Here's the drawing with two shaded views (mm, measured from the low corner). I have some questions. A direction names the side the tool comes from. Coordinates: 2 decimals unless noted, no trailing zeros. Loops run counter-clockwise (first coordinate to the right, second up) from the corner with the lowest first, then second, coordinate; pieces in that order, holes last. Notation, with made-up numbers: (11.25, 57.25) - (38.25, 57.25) arc R11 ccw to (38.25, 78.25) - close; hole circle Ø7 at (66.5, 68). An arc over 180 degrees is marked (long way). Use a Markdown table: item, result.
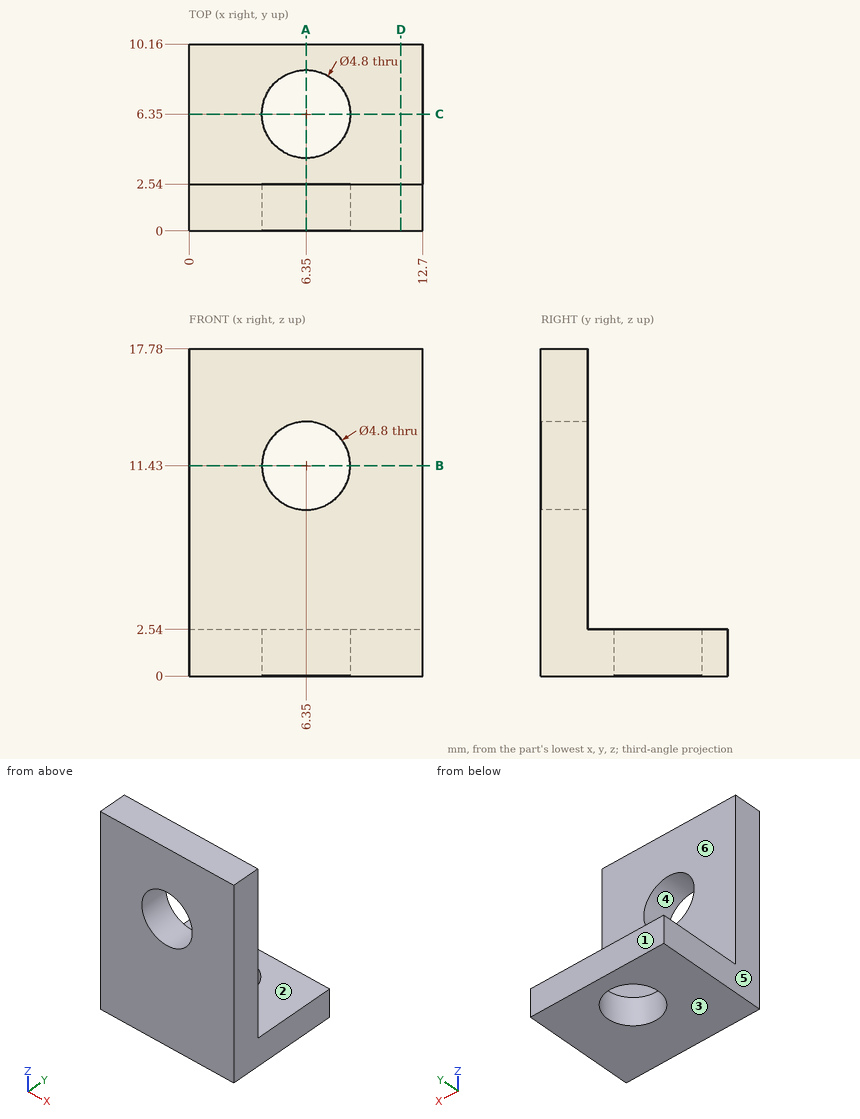
Q1. Which directions (+Z, -Z, +X, -X, +Y, -Y) give clear straight access to the entire face, cutting with the end or side of a thin tool? Please do the marked faces 5 and 6.
Check values:
| item | result |
|---|---|
| face 5 | +Z, -Z, -X, +Y, -Y |
| face 6 | +Z, +X, -X, +Y |
Q2. Please list where these lines run through material, in increasing order: L1, parallel to Y at x = 6.35, z = 1; L2, parallel to Z at x = 6.35, y = 1.2; L3, parallel to Y at x = 4.75, z = 3.75. Write a range as from..to.
Check values:
| item | result |
|---|---|
| L1 | 0..3.95, 8.75..10.16 |
| L2 | 0..9.03, 13.83..17.78 |
| L3 | 0..2.54 |
Q3. Will these pins go through, and if not, where does the flat tip stop? P1, Ø5, axis at x = 7.5, y = 7, coming from the +Z side; P2, Ø6, axis at x = 4, y = 5.5, coming from the +Z side; P3, Ø6, axis at x = 6.35, z = 11.43, coming from the +Y side.
Check values:
| item | result |
|---|---|
| P1 | z = 2.54 |
| P2 | z = 17.78 |
| P3 | y = 2.54 |
Q4. I want a section at D-D, the plane x = 11.5. Write out the boundary of the cut face in (y, z), then the cut area to 3 significant figures.
Check values:
| item | result |
|---|---|
| outline | (0, 0) - (10.16, 0) - (10.16, 2.54) - (2.54, 2.54) - (2.54, 17.78) - (0, 17.78) - close |
| area | 64.5 mm^2 |
Q5. I want a section at B-B, the plane z = 11.43. Write out the boundary of the cut face in (x, y), then the cut area to 3 significant figures.
Check values:
| item | result |
|---|---|
| outline | (0, 0) - (3.95, 0) - (3.95, 2.54) - (0, 2.54) - close; (8.75, 0) - (12.7, 0) - (12.7, 2.54) - (8.75, 2.54) - close |
| area | 20.1 mm^2 |
Q6. I want a section at A-A, the plane x = 6.35. Write out the boundary of the cut face in (y, z), then the cut area to 3 significant figures.
Check values:
| item | result |
|---|---|
| outline | (0, 0) - (3.95, 0) - (3.95, 2.54) - (2.54, 2.54) - (2.54, 9.03) - (0, 9.03) - close; (0, 13.83) - (2.54, 13.83) - (2.54, 17.78) - (0, 17.78) - close; (8.75, 0) - (10.16, 0) - (10.16, 2.54) - (8.75, 2.54) - close |
| area | 40.1 mm^2 |
Q7. If we mould it in two halves opening along Z, with no side actions, what happens to the marked faces 1, 2, 3 and 4? For each: pulls with the +Z half, pulls with the -Z half, needs draft (parallel to the pull), parting line crosses it, or undercut.
Check values:
| item | result |
|---|---|
| face 1 | needs draft |
| face 2 | pulls with the +Z half |
| face 3 | pulls with the -Z half |
| face 4 | undercut |
